For this review, take the finished solid that the model builds, in its own axes (mm). A direction names the side the tool comes from. Round coordinates to 2 decimals unless told otherwise and drop trailing zeros. Write each loop counter-clockwise with the first axis right and the second up, starting at its lowest first coordinate (ties: lowest second). Pieces come first, ordered by that corner, then holes. Notation, with made-up numbers: M 54,-6.5 L 86,-6.5 A32 cw 86,24.5 Z; hole C 2.25,-17.5 d2. An arc over 180 degrees is marked long. One line per question, with ' | ' between items.
Autodesk Inventor part; units mm, degrees
ref_plane "YZ Plane" through (0, 0, 0) normal (1, 0, 0) x (0, 1, 0)
ref_plane "XZ Plane" through (0, 0, 0) normal (0, 1, 0) x (-1, 0, 0)
ref_plane "XY Plane" through (0, 0, 0) normal (0, 0, 1) x (1, 0, 0)
sketch "Sketch1" plane through (0, 0, 0) normal (0, 1, 0) x (-1, 0, 0)
  line L0 (-20.5, 35) -> (20.5, 35)
  line L1 (20.5, 35) -> (20.5, -35)
  line L2 (20.5, -35) -> (-20.5, -35)
  line L3 (-20.5, -35) -> (-20.5, 35)
  line L4 (-20.5, 35) -> (20.5, -35) construction
  line L5 (20.5, 35) -> (-20.5, -35) construction
  line L6 (-50, 75) -> (50, 75)
  line L7 (50, 75) -> (50, -75)
  line L8 (50, -75) -> (-50, -75)
  line L9 (-50, -75) -> (-50, 75)
  line L10 (-50, 75) -> (50, -75) construction
  line L11 (50, 75) -> (-50, -75) construction
  point P0 (0, 0)
  dimension "d0" = 41
  dimension "d1" = 70
  dimension "d2" = 150
  dimension "d3" = 100
extrude "Extrusion1" add sketch "Sketch1" along normal blind 10
extrude "Extrusion2" add sketch "Sketch1" along normal blind 5 contours L0 L1 L2 L3
chamfer "Chamfer1" distance 1 angle 45 4 edges at (-20.5, 10, 0) (0, 10, 35) (0, 10, -35) (20.5, 10, 0)
chamfer "Chamfer2" distance 8 angle 45 4 edges at (-50, 5, 75) (-50, 5, -75) (50, 5, -75) (50, 5, 75)
properties part number "pallet"
Item 1: Insertion check: pin 1 Ø10 at (x, z) = (19, -17.5) entering from +Y. The pin has a flat end and moves straight along its axis. Give the tip position at first contact, or say it passes through.
Results:
pin 1: y = 10
Item 2: To check wall thickness, follow line 1 along Z through (x, y) = (8.5, 7.75); line 2 along X through (y, z) = (7.5, 31); line 3 along Z through (x, y) = (43.5, 6.75). State the ranges of each line that lie inside material, in increasing order. Write a range as from..to.
Results:
line 1: -75..-35, 35..75 | line 2: -50..-20.5, 20.5..50 | line 3: -73.5..73.5
Item 3: Take a section at B-B (x = 1). Write out the cut boundary in (y, z).
Results:
outline: M 0,-75 L 10,-75 L 10,-36 L 9,-35 L 5,-35 L 5,35 L 9,35 L 10,36 L 10,75 L 0,75 Z
Item 4: Machinability: for faces 1 (the face through (46, 5, 71)), 2 (the face through (0, 7, -35)), which of the approach directions +Z, -Z, +X, -X, +Y, -Y give a long, thin tool a straight path to every point of the face, cutting with its end or side? Answer none if there is none.
Results:
face 1: +Z, +X, +Y, -Y | face 2: +Y
Item 5: Take a section at C-C (z = 29.5). Write out the cut boundary in (x, y).
Results:
outline: M -50,0 L 50,0 L 50,10 L 21.5,10 L 20.5,9 L 20.5,5 L -20.5,5 L -20.5,9 L -21.5,10 L -50,10 Z
Item 6: Mouldability with a two-part tool opening along X and no side actions: class faces 3 (the face through (-50, 5, 1)), 4 (the face through (1, 0, 1)), 5 (the face through (20.5, 7, 0)) as +X half, -X half, draft (parallel to the pull), parting line (faces both ways), or undercut.
Results:
face 3: -X half | face 4: draft | face 5: undercut
Item 7: Take a section at A-A (y = 7.25). Write out the cut boundary in (x, z).
Results:
outline: M -50,-67 L -42,-75 L 42,-75 L 50,-67 L 50,67 L 42,75 L -42,75 L -50,67 Z; hole M -20.5,-35 L 20.5,-35 L 20.5,35 L -20.5,35 Z
